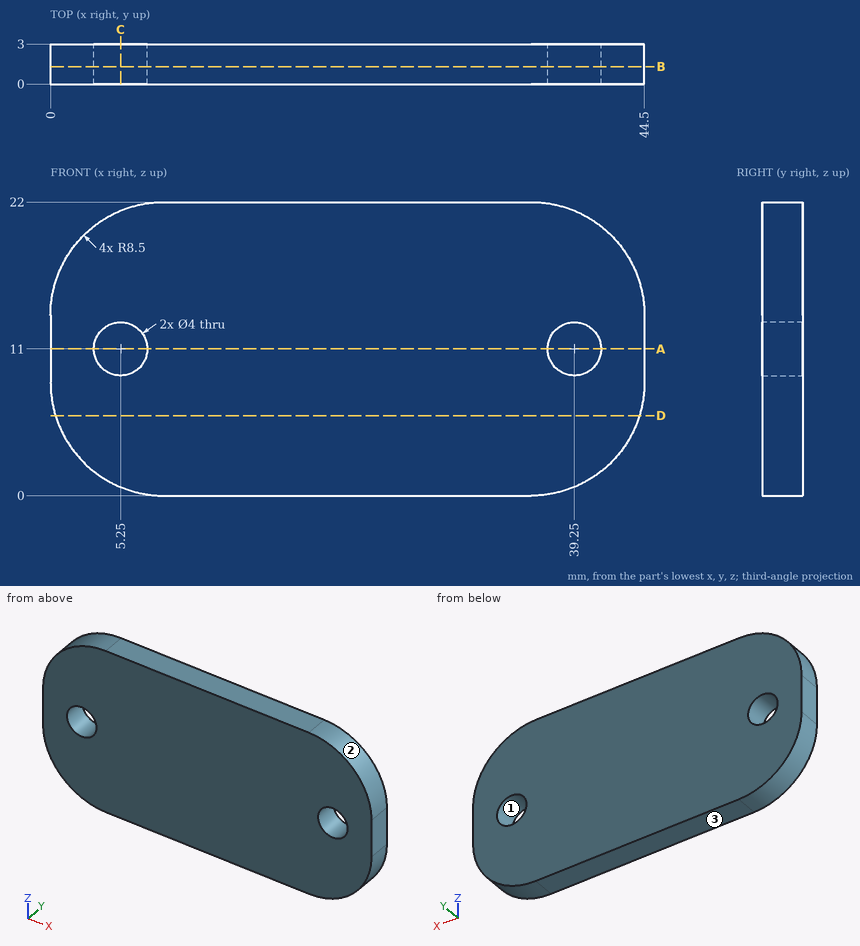
Can you work these out from the drawing? Everything is in mm from the part's minimum corner. Coordinates: 2 decimals unless noted, no trailing zeros. Loops run counter-clockwise (first coordinate to the right, second up) from the corner with the lowest first, then second, coordinate; pieces in that order, holes last.
1) Imagine slicing it at A-A on z = 11. List the corners of the cut face in (x, y) for me, plus the area to 4 significant figures.
2) I need wall thicknesses on probe 1 along X at (y, z) = (0.7, 11); probe 2 along X at (y, z) = (2.7, 10); probe 3 along X at (y, z) = (0.6, 6.5). Which ranges of each line are inside material? Lowest first, please.
3) Imagine slicing it at C-C on x = 5.25. List the corners of the cut face in (y, z) for me, plus the area to 3 significant figures.
4) Thinking about a two-plate mould opening in X: for the marked faces 1, 2 and 3, which applies, pulls with the +X half, pulls with the -X half, needs draft (parallel to the pull), parting line crosses it, or undercut?
5) Imagine slicing it at D-D on z = 6. List the corners of the cut face in (x, y) for me.
6) For pin 1 (2.5 mm diameter, centred on x = 5.25, z = 11, fed in from -Y), with a flat end and sliding along its axis, tell me the tip position at first contact or that it passes through.
7) Imagine slicing it at B-B on y = 1.3. List the corners of the cut face in (x, z) for me.
Completed:
1. outline: (0, 0) - (3.25, 0) - (3.25, 3) - (0, 3) - close; (7.25, 0) - (37.25, 0) - (37.25, 3) - (7.25, 3) - close; (41.25, 0) - (44.5, 0) - (44.5, 3) - (41.25, 3) - close
1. area: 109.5 mm2
2. probe 1: x = 0 to 3.25, 7.25 to 37.25, 41.25 to 44.5
2. probe 2: x = 0 to 3.52, 6.98 to 37.52, 40.98 to 44.5
2. probe 3: x = 0.24 to 44.26
3. outline: (0, 0.65) - (3, 0.65) - (3, 9) - (0, 9) - close; (0, 13) - (3, 13) - (3, 21.35) - (0, 21.35) - close
3. area: 50.1 mm2
4. face 1: undercut
4. face 2: pulls with the +X half
4. face 3: needs draft
5. outline: (0.38, 0) - (44.12, 0) - (44.12, 3) - (0.38, 3) - close
6. pin 1: passes through
7. outline: (0, 8.5) arc R8.5 ccw to (8.5, 0) - (36, 0) arc R8.5 ccw to (44.5, 8.5) - (44.5, 13.5) arc R8.5 ccw to (36, 22) - (8.5, 22) arc R8.5 ccw to (0, 13.5) - close; hole circle Ø4 at (5.25, 11); hole circle Ø4 at (39.25, 11)
